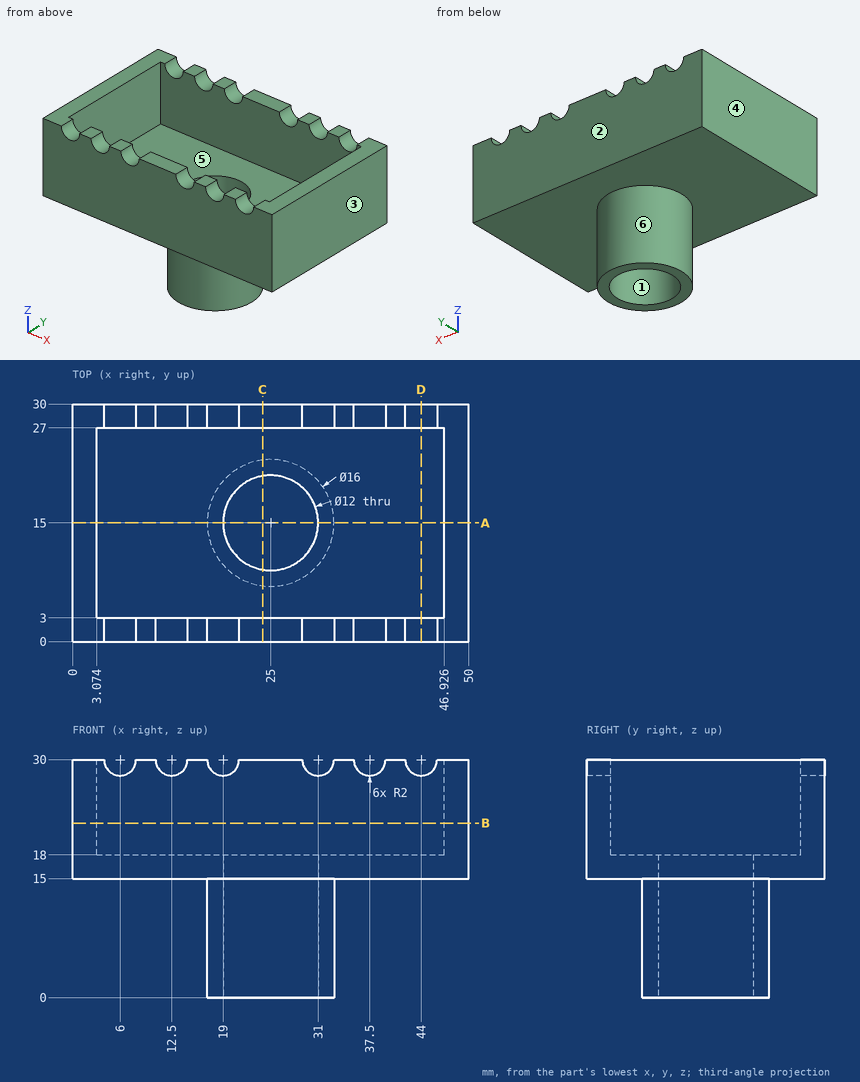
Input: dimensioned drawing with shaded views. Units: mm. Origin: part minimum x, y, z. A direction names the side the tool comes from. Coordinates: 2 decimals unless noted, no trailing zeros. Write each loop counter-clockwise with the first axis right and the second up, starting at its lowest first coordinate (ties: lowest second). Pieces come first, ordered by that corner, then holes. Notation, with made-up numbers: (41.5, 4) -> (79.5, 4) arc R6 cw to (79.5, 15) -> close; hole circle Ø5 at (-26, 56.25). An arc over 180 degrees is marked (long way). Return JSON: item names as keys, results as strings. Group by question number.
1) Set-up query: the marked faces 4, 5 and 6. Return all of +Z, -Z, +X, -X, +Y, -Y with unobstructed straight access to the full face (end or side cutting, diameter ignored); none if empty.
2) Section query B-B, the plane z = 22. Return loops of the section in (x, y).
3) Mould query, pull axis Y, two halves, no side actions, for the marked faces 1, 2 and 3. Classes: +Y half, -Y half, draft (parallel to the pull), parting line (faces both ways), or undercut.
4) Section query A-A, the plane y = 15. Return loops of the section in (x, z), plus the area to 3 significant figures.
5) Section query C-C, the plane x = 24. Return loops of the section in (y, z).
6) Section query D-D, the plane x = 44. Return loops of the section in (y, z), plus the area to 3 significant figures.
7) Ray query, line 1 along Y through (x, z) = (29, 21.75); line 2 along Y through (x, z) = (25, 5.75); line 3 along X through (y, z) = (7.25, 25.25). Return the intervals inside material, ascending.
8) Contact query for flat-ended pins moving along their axis: P1, Ø10, axis at x = 26.5, z = 7.5, coming from the -Y side; P2, Ø2, axis at y = 13.5, z = 7, coming from the +X side; P3, Ø3, axis at x = 41.5, z = 27, coming from the -Y side; P4, Ø12, axis at x = 30.5, y = 11, coming from the +Z side. Output: stop coordinate, or through.
From the geometry:
{
 "1": {"face 4": "+Z, -Z, -X, +Y, -Y", "face 5": "+Z", "face 6": "-Z"},
 "2": {"outline": "(0, 0) -> (50, 0) -> (50, 30) -> (0, 30) -> close; hole (3.07, 3) -> (46.93, 3) -> (46.93, 27) -> (3.07, 27) -> close"},
 "3": {"face 1": "undercut", "face 2": "+Y half", "face 3": "draft"},
 "4": {"outline": "(0, 15) -> (17, 15) -> (17, 0) -> (19, 0) -> (19, 18) -> (3.07, 18) -> (3.07, 30) -> (0, 30) -> close; (31, 0) -> (33, 0) -> (33, 15) -> (50, 15) -> (50, 30) -> (46.93, 30) -> (46.93, 18) -> (31, 18) -> close", "area": "248 mm²"},
 "5": {"outline": "(0, 15) -> (7.06, 15) -> (7.06, 0) -> (9.08, 0) -> (9.08, 18) -> (3, 18) -> (3, 30) -> (0, 30) -> close; (20.92, 0) -> (22.94, 0) -> (22.94, 15) -> (30, 15) -> (30, 30) -> (27, 30) -> (27, 18) -> (20.92, 18) -> close"},
 "6": {"outline": "(0, 15) -> (30, 15) -> (30, 28) -> (27, 28) -> (27, 18) -> (3, 18) -> (3, 28) -> (0, 28) -> close", "area": "150 mm²"},
 "7": {"line 1": "0 to 3, 27 to 30", "line 2": "7 to 9, 21 to 23", "line 3": "0 to 3.07, 46.93 to 50"},
 "8": {"P1": "y = 7", "P2": "x = 32.98", "P3": "y = 0", "P4": "z = 18"}
}
